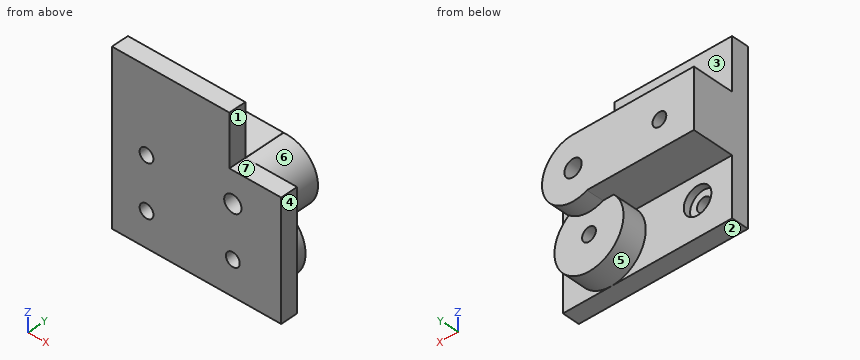
```python
from build123d import *

# Parameters (mm, degrees)
SKETCH1_R           = 2
SKETCH1_R_2         = 2.5
BOSS_EXTRUDE1_DEPTH = 5
SKETCH2_R           = 4
CUT_EXTRUDE1_DEPTH  = 2
SKETCH3_R           = 10
BOSS_EXTRUDE2_DEPTH = 12
SKETCH4_R           = 2
CUT_EXTRUDE2_DEPTH  = 12
SKETCH5_R           = 10
SKETCH5_R_2         = 2
CUT_EXTRUDE3_DEPTH  = 5
SKETCH6_R           = 9
SKETCH6_R_2         = 2.5
BOSS_EXTRUDE3_DEPTH = 12
SKETCH7_R           = 2.299679875
SKETCH7_W           = 34
SKETCH7_H           = 17.049766734
SKETCH7_R_2         = 2
BOSS_EXTRUDE4_DEPTH = 12
SKETCH9_R           = 2.5
CUT_EXTRUDE5_DEPTH  = 27


with BuildPart() as part:
    # Sketch1 → Boss-Extrude1 (new body)
    with BuildSketch(Plane(origin=(0, 0, 0), x_dir=(1, 0, 0), z_dir=(0, 1, 0))):
        Polygon((0, 49), (0, 0), (34, 0), (34, 15), (49, 15), (49, 49), align=None)
        with Locations((10, 24)):
            Circle(SKETCH1_R, mode=Mode.SUBTRACT)
        with Locations((35, 24)):
            Circle(SKETCH1_R_2, mode=Mode.SUBTRACT)
        with Locations((10, 39)):
            Circle(SKETCH1_R, mode=Mode.SUBTRACT)
        with Locations((35, 39)):
            Circle(SKETCH1_R, mode=Mode.SUBTRACT)
    extrude(amount=BOSS_EXTRUDE1_DEPTH)

    # Sketch2 → Cut-Extrude1 (cut)
    with BuildSketch(Plane(origin=(0, 5, 0), x_dir=(1, 0, 0), z_dir=(0, 1, 0))):
        with Locations((10, 39)):
            Circle(SKETCH2_R)
    extrude(amount=-CUT_EXTRUDE1_DEPTH, mode=Mode.SUBTRACT)

    # Sketch3 → Boss-Extrude2 (add)
    with BuildSketch(Plane(origin=(0, 5, 0), x_dir=(1, 0, 0), z_dir=(0, 1, 0))):
        with Locations((35, 39)):
            Circle(SKETCH3_R)
    extrude(amount=BOSS_EXTRUDE2_DEPTH)

    # Sketch4 → Cut-Extrude2 (cut)
    with BuildSketch(Plane.XZ.offset(-5)):
        with Locations((35, -39)):
            Circle(SKETCH4_R)
    extrude(amount=-CUT_EXTRUDE2_DEPTH, mode=Mode.SUBTRACT)

    # Sketch5 → Cut-Extrude3 (cut)
    with BuildSketch(Plane(origin=(0, 17, 0), x_dir=(1, 0, 0), z_dir=(0, 1, 0))):
        with Locations((35, 39)):
            Circle(SKETCH5_R)
        with Locations((35, 39)):
            Circle(SKETCH5_R_2, mode=Mode.SUBTRACT)
    extrude(amount=-CUT_EXTRUDE3_DEPTH, mode=Mode.SUBTRACT)

    # Sketch6 → Boss-Extrude3 (add)
    with BuildSketch(Plane(origin=(0, 5, 0), x_dir=(1, 0, 0), z_dir=(0, 1, 0))):
        with Locations((35, 24)):
            Circle(SKETCH6_R)
        with Locations((35, 24)):
            Circle(SKETCH6_R_2, mode=Mode.SUBTRACT)
    extrude(amount=BOSS_EXTRUDE3_DEPTH)

    # Sketch7 → Boss-Extrude4 (add)
    with BuildSketch(Plane(origin=(0, 5, 0), x_dir=(1, 0, 0), z_dir=(0, 1, 0))):
        with Locations((35, 24)):
            Circle(SKETCH7_R)
        with Locations((17, 23.524883367)):
            Rectangle(SKETCH7_W, SKETCH7_H)
        with Locations((10, 24)):
            Circle(SKETCH7_R_2, mode=Mode.SUBTRACT)
    extrude(amount=BOSS_EXTRUDE4_DEPTH)

    # Sketch9 → Cut-Extrude5 (cut)
    with BuildSketch(Plane(origin=(0, 17, 0), x_dir=(1, 0, 0), z_dir=(0, 1, 0))):
        with Locations((35, 24)):
            Circle(SKETCH9_R)
    extrude(amount=-CUT_EXTRUDE5_DEPTH, mode=Mode.SUBTRACT)


solid = part.part
```
The model under review builds one solid part; all positions refer to its coordinate system, in mm. Face numbers are marked on the shaded views. A direction names the side the tool comes from. Round coordinates to 2 decimals unless told otherwise and drop trailing zeros. Order: outer loops, then holes, each group sorted by start corner. A loop starts at its lowest first (then second) coordinate and runs counter-clockwise, first axis right, second up.
(1) Take a section at A-A, the plane x = 10. State the section outline as (y, z) points, plus the area to 3 significant figures.
Working result:
outline: (0, -49) - (5, -49) - (5, -43) - (3, -43) - (3, -41) - (0, -41) - close; (0, -37) - (3, -37) - (3, -35) - (5, -35) - (5, -32.05) - (17, -32.05) - (17, -26) - (0, -26) - close; (0, -22) - (17, -22) - (17, -15) - (5, -15) - (5, 0) - (0, 0) - close
area: 354 mm2
(2) Wall thickness on L1, parallel to Z at x = 10, y = 4.25; L2, parallel to Z at x = 35, y = 2.5; L3, parallel to X at y = 2.15, z = -39: over which ranges is each line inside the solid? List them lowest first.
Working result:
L1: z = -49 to -43, -35 to -26, -22 to 0
L2: z = -49 to -41, -37 to -26.5, -21.5 to -15
L3: x = 0 to 8, 12 to 33, 37 to 49
(3) For P1, Ø6, axis at x = 21.5, y = 12.5, coming from the -Z side; P2, Ø2.5, axis at x = 11.5, z = -39.5, coming from the +Y side; P3, Ø4, axis at x = 40.5, y = 3.5, coming from the +Z side, all flat-tipped, find the tip position at first contact; note any pin that passes through.
Working result:
P1: stops at z = -32.05
P2: stops at y = 3
P3: stops at z = -15
(4) Take a section at C-C, the plane z = -39. State the section outline as (x, y) points, plus the area to 3 significant figures.
Working result:
outline: (0, 0) - (8, 0) - (8, 3) - (6, 3) - (6, 5) - (0, 5) - close; (12, 0) - (33, 0) - (33, 12) - (25, 12) - (25, 5) - (14, 5) - (14, 3) - (12, 3) - close; (37, 0) - (49, 0) - (49, 5) - (45, 5) - (45, 12) - (37, 12) - close
area: 309 mm2
(5) Mouldability with a two-part tool opening along Z and no side actions: class the marked faces 4, 5, 6 and 7 as released by +Z, released by -Z, zero draft, split by the parting line, or undercut.
Working result:
face 4: zero draft
face 5: undercut
face 6: undercut
face 7: released by +Z
(6) Take a section at D-D, the plane y = 16. State the section outline as (x, z) points.
Working result:
outline: (0, -32.05) - (30.97, -32.05) arc R9 ccw (long way) to (34, -15.06) - (34, -15) - (0, -15) - close; hole circle Ø4 at (10, -24); hole circle Ø5 at (35, -24)
(7) Tool access review of the marked faces 1, 2 and 3: name each direction out of +Z, -Z, +X, -X, +Y, -Y from which nothing blocks a thin tool from reaching the whole face with its end or side.
Working result:
face 1: +Z, +X, +Y, -Y
face 2: -Z, +X, -X, +Y, -Y
face 3: +Z, +X, -X, +Y
(8) Take a section at B-B, the plane y = 4. State the section outline as (x, z) points, plus the area to 3 significant figures.
Working result:
outline: (0, -49) - (49, -49) - (49, -15) - (34, -15) - (34, 0) - (0, 0) - close; hole circle Ø8 at (10, -39); hole circle Ø4 at (10, -24); hole circle Ø5 at (35, -24); hole circle Ø4 at (35, -39)
area: 2,080 mm2
